Answer from the drawing. Dimensions are ordinates in mm from the lowest x, y and z of the part. A direction names the side the tool comes from. Round coordinates to 2 decimals unless told otherwise and drop trailing zeros. Write each loop counter-clockwise with the first axis right and the second up, starting at its lowest first coordinate (ties: lowest second). Pieces come first, ordered by that corner, then holes. Notation, with made-up numbers: (10, 57) -> (66, 57) arc R18 cw to (66, 73) -> close; hole circle Ø11 at (-27.5, -15.5). An arc over 180 degrees is marked (long way). Answer as a JSON object with one key per item and string values. Group by question number.
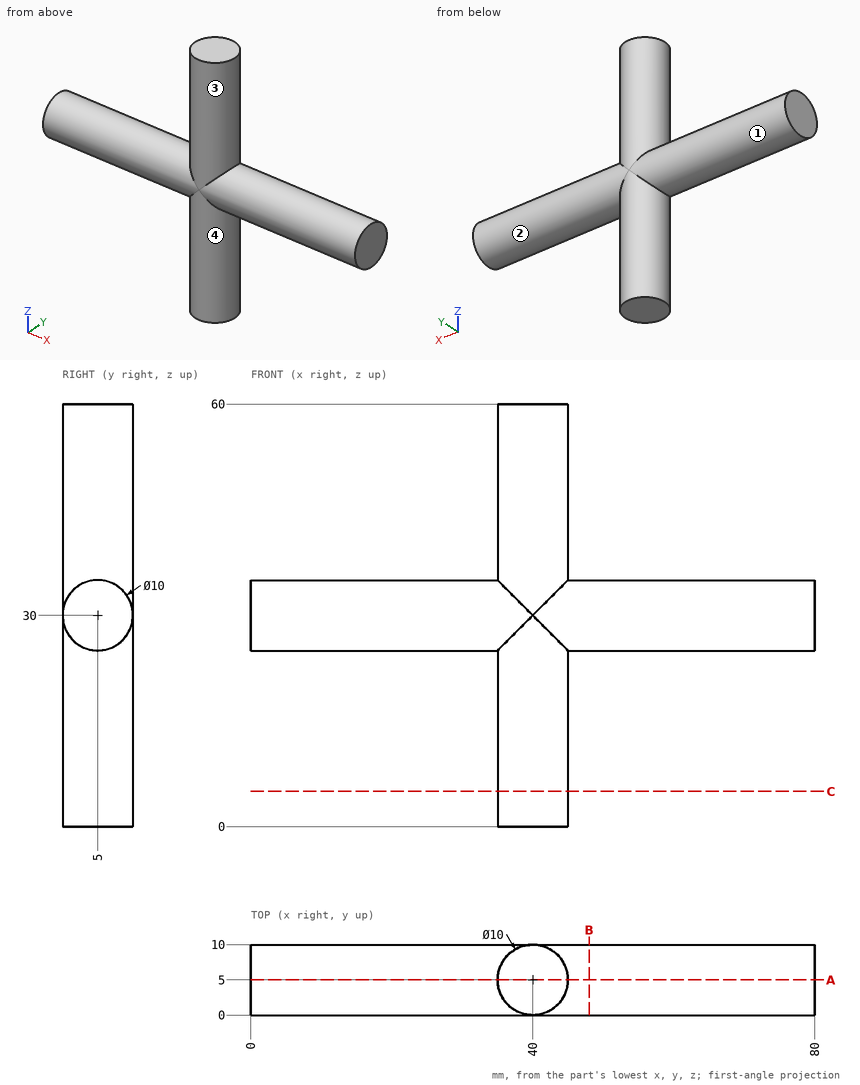
1) A tool of negligible diameter and unlimited length cuts with its end or side. For the marked faces 1, 2, 3 and 4, from which of +Z, -Z, +X, -X, +Y, -Y can it reach the whole face along a straight path? Write none if from no direction.
2) A cutting plane is placed at C-C on z = 5. Determine the outline of the cut face in (x, y), plus the area to 3 significant figures.
3) A cutting plane is placed at B-B on x = 48. Determine the outline of the cut face in (y, z).
4) Each of these flat-tipped pins is pushed along its axis until it touches: P1, Ø1, axis at y = 5, z = 43, coming from the -X side; P2, Ø1, axis at x = 42, z = 22, coming from the +Y side; P3, Ø5, axis at x = 62.5, y = 8, coming from the -Z side. Where does it stop, or does it pass through?
5) A cutting plane is placed at A-A on y = 5. Determine the outline of the cut face in (x, z), plus the area to 3 significant figures.
6) Straight lines are drawn through the part: L1, parallel to X at y = 4.75, z = 46; L2, parallel to Z at x = 21.5, y = 2.75; L3, parallel to Z at x = 48, y = 6.75. For each, find the intervals that lie inside material, in ascending order.
Established:
{
 "1": {"face 1": "-X", "face 2": "+X", "face 3": "+Z", "face 4": "-Z"},
 "2": {"outline": "circle Ø10 at (40, 5)", "area": "78.5 mm²"},
 "3": {"outline": "circle Ø10 at (5, 30)"},
 "4": {"P1": "stops at x = 35", "P2": "stops at y = 9.77", "P3": "stops at z = 25.03"},
 "5": {"outline": "(0, 25) -> (35, 25) -> (35, 0) -> (45, 0) -> (45, 25) -> (80, 25) -> (80, 35) -> (45, 35) -> (45, 60) -> (35, 60) -> (35, 35) -> (0, 35) -> close", "area": "1,300 mm²"},
 "6": {"L1": "x = 35.01 to 44.99", "L2": "z = 25.53 to 34.47", "L3": "z = 25.32 to 34.68"}
}
